Autodesk Inventor part; units mm, degrees
ref_plane "YZ Plane" through (0, 0, 0) normal (1, 0, 0) x (0, 1, 0)
ref_plane "XZ Plane" through (0, 0, 0) normal (0, 1, 0) x (-1, 0, 0)
ref_plane "XY Plane" through (0, 0, 0) normal (0, 0, 1) x (1, 0, 0)
sketch "Sketch1" plane through (0, 0, 0) normal (0, 0, 1) x (1, 0, 0)
  line L0 (-166.4634, 98.1707) -> (205.1366, 98.1707)
  line L1 (205.1366, 98.1707) -> (205.1366, -171.8293)
  line L2 (205.1366, -171.8293) -> (-166.4634, -171.8293)
  line L3 (-166.4634, -171.8293) -> (-166.4634, 98.1707)
  point P0 (0, 0)
  dimension "d0" = 371.6
  dimension "d1" = 270
extrude "Extrusion1" add sketch "Sketch1" along normal blind 6
fillet "Fillet1" radius 2 1 edges at (-166.4634, 98.1707, 3)
fillet "Fillet2" radius 2 3 edges at (205.1366, 98.1707, 3) (205.1366, -171.8293, 3) (-166.4634, -171.8293, 3)
sketch "Sketch2" plane through (0, 0, 6) normal (0, 0, 1) x (1, 0, 0)
  line L0 (200.1366, -161.8293) -> (140.1366, -161.8293)
  line L1 (140.1366, -161.8293) -> (140.1366, 88.1707)
  line L2 (140.1366, 88.1707) -> (200.1366, 88.1707)
  line L3 (200.1366, 88.1707) -> (200.1366, -161.8293)
  line L4 (-101.4634, -161.8293) -> (-161.4634, -161.8293)
  line L5 (-161.4634, -161.8293) -> (-161.4634, 88.1707)
  line L6 (-161.4634, 88.1707) -> (-101.4634, 88.1707)
  line L7 (-101.4634, 88.1707) -> (-101.4634, -161.8293)
  line L8 (205.1366, -169.8293) -> (205.1366, 96.1707)
  line L9 (203.1366, 98.1707) -> (-164.4634, 98.1707)
  line L10 (-166.4634, 96.1707) -> (-166.4634, -169.8293)
  point P0 (0, 0)
  dimension "d6" = 60
  dimension "d7" = 60
  dimension "d8" = 250
  dimension "d9" = 250
  dimension "d10" = 65
  dimension "d11" = 10
  dimension "d12" = 10
  dimension "d13" = 65
extrude "Extrusion2" cut sketch "Sketch2" against normal through all
fillet "Fillet3" radius 2 8 edges at (200.1366, -161.8293, 3) (-101.4634, -161.8293, 3) (-161.4634, -161.8293, 3) (140.1366, -161.8293, 3) (200.1366, 88.1707, 3) (-101.4634, 88.1707, 3) (-161.4634, 88.1707, 3) (140.1366, 88.1707, 3)
sketch "Sketch3" plane through (0, 0, 6) normal (0, 0, 1) x (1, 0, 0)
  circle A0 centre (-91.4634, 58.1707) radius 4.7928
  circle A1 centre (-51.4634, 58.1707) radius 10.8449
  circle A2 centre (-11.4634, 58.1707) radius 12.4429
  circle A3 centre (50.1366, 58.1707) radius 12.4797
  circle A4 centre (90.1366, 58.1707) radius 18.3008
  circle A5 centre (130.1366, 58.1707) radius 8.1337
  circle A6 centre (-91.4634, -1.8293) radius 12.8783
  circle A7 centre (-51.4634, -1.8293) radius 10.8449
  circle A8 centre (-11.4634, -1.8293) radius 12.4429
  circle A9 centre (50.1366, -1.8293) radius 10.8449
  circle A10 centre (90.1366, -1.8293) radius 10.1671
  circle A11 centre (130.1366, -1.8293) radius 18.5005
  line L0 (-101.4634, 86.1707) -> (-101.4634, -159.8293)
  line L1 (140.1366, -159.8293) -> (140.1366, 86.1707)
  line L2 (-159.4634, 88.1707) -> (-103.4634, 88.1707)
  line L3 (142.1366, 88.1707) -> (198.1366, 88.1707)
  circle A12 centre (-91.4634, -71.8293) radius 15.1871
  circle A13 centre (-91.4634, -131.8293) radius 15.3472
  circle A14 centre (-51.4634, -131.8293) radius 18.7949
  circle A15 centre (-51.4634, -71.8293) radius 21.2619
  circle A16 centre (-11.4634, -71.8293) radius 19.027
  circle A17 centre (-11.4634, -131.8293) radius 15.2356
  circle A18 centre (50.1366, -71.8293) radius 22.218
  circle A19 centre (50.1366, -131.8293) radius 15.9181
  circle A20 centre (90.1366, -71.8293) radius 11.5297
  circle A21 centre (130.1366, -71.8293) radius 12.0044
  circle A22 centre (90.1366, -131.8293) radius 9.1325
  circle A23 centre (130.1366, -131.8293) radius 9.1929
  line L4 (-164.4634, -171.8293) -> (203.1366, -171.8293)
  line L5 (-103.4634, -161.8293) -> (-159.4634, -161.8293)
  line L6 (198.1366, -161.8293) -> (142.1366, -161.8293)
  point P0 (0, 0)
  point P1 (140.1366, 86.1707)
  point P2 (-101.4634, -171.8293)
  point P3 (168.5366, -171.8293)
  dimension "d17" = 10
  dimension "d18" = 40
  dimension "d19" = 40
  dimension "d20" = 10
  dimension "d22" = 40
  dimension "d23" = 40
  dimension "d24" = 30
  dimension "d25" = 30
  dimension "d26" = 30
  dimension "d27" = 30
  dimension "d28" = 30
  dimension "d29" = 30
  dimension "d30" = 60
  dimension "d31" = 10
  dimension "d32" = 60
  dimension "d33" = 60
  dimension "d34" = 40
  dimension "d35" = 40
  dimension "d36" = 40
  dimension "d37" = 40
  dimension "d38" = 10
  dimension "d39" = 60
  dimension "d40" = 60
  dimension "d41" = 60
  dimension "d42" = 10
  dimension "d43" = 10
  dimension "d45" = 60
  dimension "d46" = 40
  dimension "d47" = 40
  dimension "d48" = 40
  dimension "d49" = 40
  dimension "d50" = 10
  dimension "d51" = 10
  dimension "d52" = 40
  dimension "d53" = 40
  dimension "d54" = 40
  dimension "d55" = 40
  dimension "d56" = 30
  dimension "d57" = 60
  dimension "d58" = 60
  dimension "d59" = 60
  dimension "d60" = 60
  dimension "d61" = 60
  dimension "d62" = 30
  dimension "d63" = 30
  dimension "d64" = 30
  dimension "d65" = 30
  dimension "d66" = 30
hole "Hole1" at (50.1366, -71.8293, 6) at (-91.4634, 58.1707, 6) at (-51.4634, 58.1707, 6) at (-11.4634, 58.1707, 6) at (-91.4634, -1.8293, 6) at (-51.4634, -1.8293, 6) at (-11.4634, -1.8293, 6) at (50.1366, -1.8293, 6) at (50.1366, 58.1707, 6) at (90.1366, 58.1707, 6) at (130.1366, 58.1707, 6) at (90.1366, -1.8293, 6) at (130.1366, -1.8293, 6) at (90.1366, -71.8293, 6) at (130.1366, -71.8293, 6) at (130.1366, -131.8293, 6) at (90.1366, -131.8293, 6) at (50.1366, -131.8293, 6) at (-91.4634, -71.8293, 6) at (-51.4634, -71.8293, 6) at (-11.4634, -71.8293, 6) at (-11.4634, -131.8293, 6) at (-51.4634, -131.8293, 6) at (-91.4634, -131.8293, 6) direction (0, 0, -1) diameter 3.3 end through all
sketch "Sketch4" plane through (0, 0, 6) normal (0, 0, 1) x (1, 0, 0)
  circle A0 centre (-91.4634, 88.1707) radius 1.5
  circle A1 centre (130.1366, 88.1707) radius 1.5
  circle A2 centre (130.1366, -161.8293) radius 1.5597
  circle A3 centre (-91.4634, -161.8293) radius 2.8966
  line L0 (203.1366, 98.1707) -> (-164.4634, 98.1707)
  line L1 (-101.4634, 86.1707) -> (-101.4634, -159.8293)
  line L2 (140.1366, -159.8293) -> (140.1366, 86.1707)
  line L3 (-164.4634, -171.8293) -> (203.1366, -171.8293)
  point P0 (0, 0)
  dimension "d74" = 3
  dimension "d75" = 10
  dimension "d76" = 10
  dimension "d77" = 10
  dimension "d78" = 3
  dimension "d79" = 10
  dimension "d80" = 10
  dimension "d81" = 10
  dimension "d82" = 10
  dimension "d83" = 10
hole "Hole2" at (-91.4634, -161.8293, 6) at (130.1366, -161.8293, 6) at (-91.4634, 88.1707, 6) at (130.1366, 88.1707, 6) direction (0, 0, -1) diameter 3 end through all
properties part number "Chassis"
Design review of the part built by this model. Coordinates are the model's own, in mm. Coordinates: 2 decimals unless noted, no trailing zeros. Order: outer loops, then holes, each group sorted by start corner. A loop starts at its lowest first (then second) coordinate and runs counter-clockwise, first axis right, second up. Notation, with made-up numbers: (43.25, -6) - (48.25, -6) arc R27 cw to (48.25, 21) - close; hole circle Ø7 at (48, 60). An arc over 180 degrees is marked (long way). Answer in a Markdown table with one row per item.
(1) Wall thickness on line 1 along X through (y, z) = (26, 3.3); line 2 along Y through (x, z) = (-148.5, 3.3): over which ranges is each line inside the solid? List them lowest first. Write a range as from..to.
Checked values:
| item | result |
|---|---|
| line 1 | -166.46..-161.46, -101.46..140.14, 200.14..205.14 |
| line 2 | -171.83..-161.83, 88.17..98.17 |
(2) Consider section C-C on z = 3.35. Give the number of separate pieces and of enclosed holes in the cut face, plus the area to 3 significant figures.
Checked values:
| item | result |
|---|---|
| separate pieces | 1 |
| enclosed holes | 30 |
| area | 70,100 mm^2 |
(3) Consider section A-A on x = -108. State the section outline as (y, z) points, plus the area to 3 significant figures.
Checked values:
| item | result |
|---|---|
| outline | (-171.83, 0) - (-161.83, 0) - (-161.83, 6) - (-171.83, 6) - close; (88.17, 0) - (98.17, 0) - (98.17, 6) - (88.17, 6) - close |
| area | 120 mm^2 |
(4) Consider section B-B on y = -30. State the section outline as (x, z) points, plus the area to 3 significant figures.
Checked values:
| item | result |
|---|---|
| outline | (-166.46, 0) - (-161.46, 0) - (-161.46, 6) - (-166.46, 6) - close; (-101.46, 0) - (140.14, 0) - (140.14, 6) - (-101.46, 6) - close; (200.14, 0) - (205.14, 0) - (205.14, 6) - (200.14, 6) - close |
| area | 1,510 mm^2 |
